Model file for the job. Use its own axes, mm. Face numbers are marked on the shaded views. Round coordinates to 2 decimals unless told otherwise and drop trailing zeros. Order: outer loops, then holes, each group sorted by start corner. A loop starts at its lowest first (then second) coordinate and runs counter-clockwise, first axis right, second up. Notation, with made-up numbers: (58.5, 22) - (63.5, 22) arc R16 ccw to (63.5, 45) - close; hole circle Ø5 at (40, 7.25). An arc over 180 degrees is marked (long way). Put each result on its own line as item: value. Start each with the question number.
Item 1: Probe probe 1 along X at (y, z) = (-29.75, 0); probe 2 along Z at (x, y) = (-10.5, -30); probe 3 along Y at (x, z) = (-11, -1.5). List the from-to ranges inside material, lowest first.
Item 2: Mould opens along Z. For the marked faces 1, 2 and 3 say: pulls with the +Z half, pulls with the -Z half, needs draft (parallel to the pull), parting line crosses it, or undercut.
Item 3: Pin check, flat tip, straight feed: pin 1 Ø2 at (y, z) = (-41.5, 2) entering from +X. Stop position of the tip, or through.
Item 4: Saw through at A-A on y = -39. List the corners of the cut face in (x, z), plus the area to 3 significant figures.
Item 5: Saw through at B-B on z = 0. List the corners of the cut face in (x, y), plus the area to 3 significant figures.
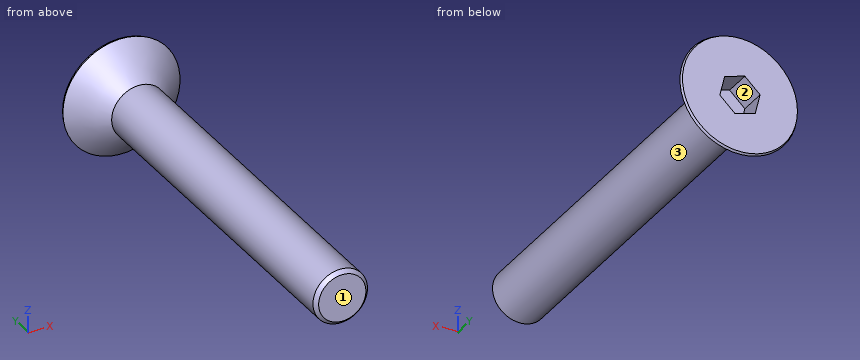
Autodesk Inventor part; units mm, degrees
ref_plane "YZ Plane" through (0, 0, 0) normal (1, 0, 0) x (0, 1, 0)
ref_plane "XZ Plane" through (0, 0, 0) normal (0, 1, 0) x (-1, 0, 0)
ref_plane "XY Plane" through (0, 0, 0) normal (0, 0, 1) x (1, 0, 0)
sketch "Sketch1" plane through (0, 0, 0) normal (0, 0, 1) x (1, 0, 0)
  line L0 (-13.7828, -22.52) -> (-10.4228, -22.52)
  line L1 (-10.4228, -22.52) -> (-10.4228, -29.38)
  line L2 (-10.4228, -29.38) -> (-10.4228, -44.38)
  line L3 (-10.4228, -44.38) -> (-11.9228, -44.38)
  line L4 (-11.9228, -44.38) -> (-11.9228, -24.38)
  line L5 (-11.9228, -24.38) -> (-13.7828, -22.52)
  point P0 (0, 0)
  dimension "d3" = 1.5
  dimension "d15" = 1.86
  dimension "d16" = 3.36
  dimension "d23" = 20
  dimension "d24" = 21.86
revolve "Revolution1" add sketch "Sketch1" angle 360 about axis through (-10.4228, -29.38, 0) along (0, -1, 0)
chamfer "Chamfer2" distance 0.2 angle 45 1 edges at (-8.9228, -44.38, 0)
chamfer "Chaflán3" distance 0.2 angle 45 1 edges at (-7.0628, -22.52, 0)
sketch "Boceto2" plane through (-10.4228, -22.52, 0) normal (0, 1, 0) x (1, 0, 0)
  line L0 (-0.8371, 0.7954) -> (0.2703, 1.1226)
  line L1 (0.2703, 1.1226) -> (1.1074, 0.3272)
  line L2 (1.1074, 0.3272) -> (0.8371, -0.7954)
  line L3 (0.8371, -0.7954) -> (-0.2703, -1.1226)
  line L4 (-0.2703, -1.1226) -> (-1.1074, -0.3272)
  line L5 (-1.1074, -0.3272) -> (-0.8371, 0.7954)
  point P0 (10.4228, 0)
  point P1 (0, 0)
  dimension "d20" = 2
extrude "Extrusión1" cut sketch "Boceto2" against normal blind 1.5
thread "Thread2"
properties part number "Tornillo Allen cabeza fresada M3x20mm"
Results found:
1. probe 1: x = -11.92 to -8.92
1. probe 2: z = -1.5 to 1.5
1. probe 3: y = -24.27 to -22.52
2. face 1: needs draft
2. face 2: undercut
2. face 3: parting line crosses it
3. pin 1: stops at x = -9.3
4. outline: circle Ø3 at (-10.42, 0)
4. area: 7.07 mm²
5. outline: (-13.64, -22.66) - (-11.92, -24.38) - (-11.92, -44.18) - (-11.72, -44.38) - (-9.12, -44.38) - (-8.92, -44.18) - (-8.92, -24.38) - (-7.2, -22.66) - (-7.26, -22.52) - (-9.39, -22.52) - (-9.39, -24.02) - (-11.45, -24.02) - (-11.45, -22.52) - (-13.58, -22.52) - close
5. area: 65.9 mm²
